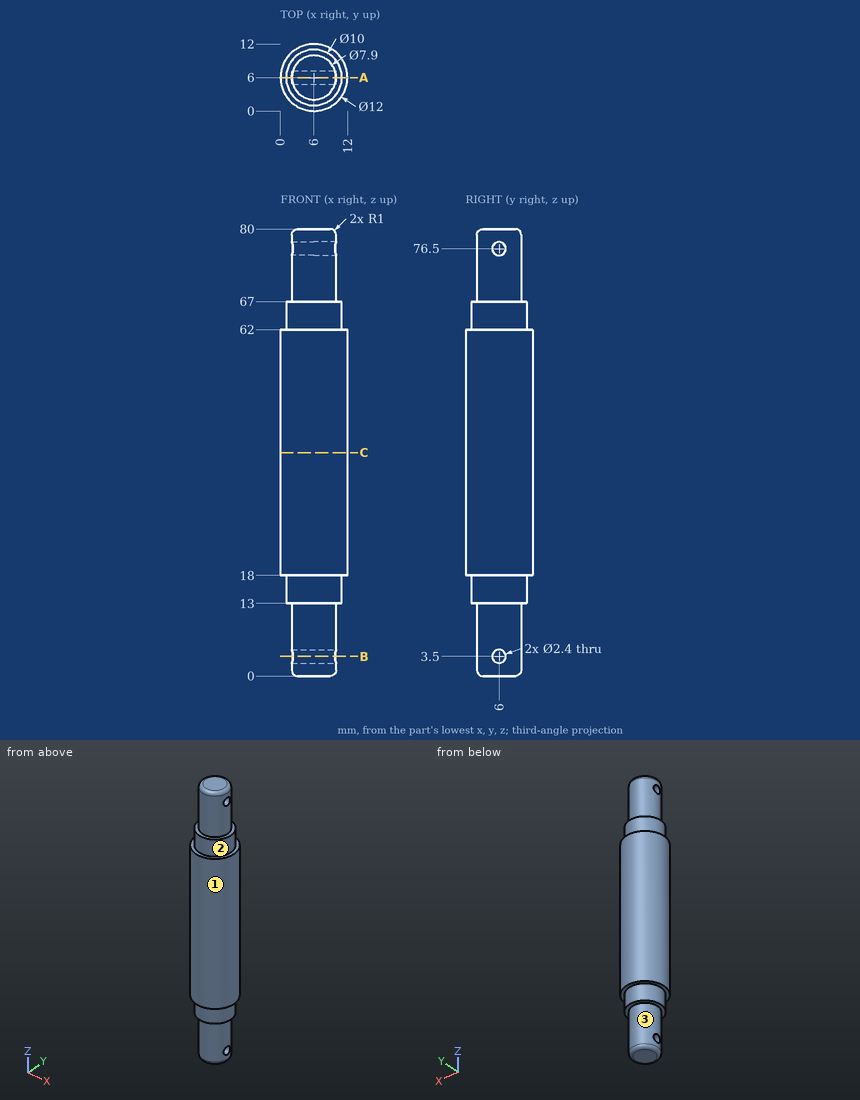
Can you work these out from the drawing? Everything is in mm from the part's minimum corner. A direction names the side the tool comes from. Coordinates: 2 decimals unless noted, no trailing zeros. Order: outer loops, then holes, each group sorted by start corner. A loop starts at its lowest first (then second) coordinate and runs counter-clockwise, first axis right, second up. Notation, with made-up numbers: M 63.25,69.25 L 105.25,69.25 A11 ccw 105.25,77.25 Z; hole C 73,-3.5 d4. An arc over 180 degrees is marked long. Answer as CSV lines item,"result". Start each with the question number.
1. On a 3-axis mill with a long thin cutter (end or side, diameter ignored), from which of +Z, -Z, +X, -X, +Y, -Y can I reach the whole of each face in a straight line? I mean the marked faces 1, 2 and 3. Say none if no direction works.
2. I want a section at A-A, the plane y = 6. Count the separate pieces of the cut face and the enclosed holes in it, and give its area (3 significant figures).
3. For pin 1 (3 mm diameter, centred on y = 6, z = 76.5, fed in from -X); pin 2 (4 mm diameter, centred on y = 6, z = 3.5, fed in from +X); pin 3 (2 mm diameter, centred on y = 10.5, z = 45.5, fed in from +X); pin 4 (5 mm diameter, centred on y = 4, z = 61, fed in from -X), each with a flat end and sliding along its axis, tell me the tip position at first contact or that it passes through.
4. I want a section at B-B, the plane z = 3.5. Write out the boundary of the cut face in (x, y), and give its area (3 significant figures).
5. I want a section at C-C, the plane z = 40. Write out the boundary of the cut face in (x, y).
6. I need wall thicknesses on line 1 (Z direction, x = 7.25, y = 6); line 2 (Y direction, x = 5.75, z = 3.5); line 3 (Z direction, x = 7.5, y = 7). Which ranges of each line are inside material? Lowest first, please. Write a range as [from, to].
Recorded:
1,face 1,"+Z, -Z"
1,face 2,"+Z"
1,face 3,"-Z"
2,separate pieces,"3"
2,enclosed holes,"0"
2,area,"795 mm2"
3,pin 1,"stops at x = 2.05"
3,pin 2,"stops at x = 9.95"
3,pin 3,"stops at x = 10.87"
3,pin 4,"stops at x = 0"
4,outline,"M 2.24,4.8 A3.95 ccw 9.76,4.8 Z; M 2.24,7.2 L 9.76,7.2 A3.95 ccw Z"
4,area,"30.4 mm2"
5,outline,"C 6,6 d12"
6,line 1,"z = [0, 2.3], [4.7, 75.3], [77.7, 80]"
6,line 2,"y = [2.06, 4.8], [7.2, 9.94]"
6,line 3,"z = [0, 2.84], [4.16, 75.84], [77.16, 80]"
